```python
from build123d import *

# Parameters (mm, degrees)
F2_R     = 4.7625
F3_DEPTH = 9.525
F4_R     = 1.5875
F5_DEPTH = 20.9169


with BuildPart() as f1:
    # F0 (on Front) → F1 (revolve)
    with BuildSketch(Plane.XZ):
        with BuildLine():
            Line((0, 33.02), (0, 0))
            add(Edge.make_bspline(
                [(9.9140361241, 6.2119723298), (5.3911280841, 4.3766633401), (5.9293914696, 2.4382627623), (0, 0)],
                knots=[0.8288382909, 0.8288382909, 0.8288382909, 0.8288382909, 1, 1, 1, 1], degree=3))
            Line((9.9140361241, 6.2119723298), (9.9140361241, 13.9279487485))
            Line((9.9140361241, 13.9279487485), (9.9140361241, 21.6439251673))
            add(Edge.make_bspline(
                [(10.16, 28.857588768), (11.523254674, 26.9400200202), (10.1686139157, 23.2379404383), (9.2103585852, 22.1157759581), (9.9140361241, 21.6439251673)],
                knots=[0.1658124621, 0.1658124621, 0.1658124621, 0.1658124621, 0.2850146806, 0.3472062164, 0.3472062164, 0.3472062164, 0.3472062164], degree=3))
            add(Edge.make_bspline(
                [(0.6915654728, 33.02), (3.173352175, 32.8639093886), (8.4465738437, 31.2677125048), (10.16, 28.857588768)],
                knots=[0.0159914469, 0.0159914469, 0.0159914469, 0.0159914469, 0.1658124621, 0.1658124621, 0.1658124621, 0.1658124621], degree=3))
            Line((0.6915654728, 33.02), (0, 33.02))
        make_face()
        with BuildLine():
            Line((10.16, 33.02), (0.6915654728, 33.02))
            add(Edge.make_bspline(
                [(0.6915654728, 33.02), (3.173352175, 32.8639093886), (8.4465738437, 31.2677125048), (10.16, 28.857588768)],
                knots=[0.0159914469, 0.0159914469, 0.0159914469, 0.0159914469, 0.1658124621, 0.1658124621, 0.1658124621, 0.1658124621], degree=3))
            Line((10.16, 28.857588768), (10.16, 33.02))
        make_face()
        with BuildLine():
            Line((9.9140361241, 13.9279487485), (9.9140361241, 6.2119723298))
            add(Edge.make_bspline(
                [(31.75, 13.483504906), (30.91482321, 10.9141221863), (15.9329484904, 8.6543310681), (9.9140361241, 6.2119723298)],
                knots=[0.60106286, 0.60106286, 0.60106286, 0.60106286, 0.8288382909, 0.8288382909, 0.8288382909, 0.8288382909], degree=3))
            Line((31.75, 13.483504906), (31.75, 13.9279487485))
            Line((31.75, 13.9279487485), (9.9140361241, 13.9279487485))
        make_face()
        with BuildLine():
            Line((9.9140361241, 21.6439251673), (9.9140361241, 13.9279487485))
            Line((9.9140361241, 13.9279487485), (31.75, 13.9279487485))
            add(Edge.make_bspline(
                [(9.9140361241, 21.6439251673), (12.6387933507, 19.8168399172), (30.8403124733, 16.6836184602), (31.75, 13.9279487485)],
                knots=[0.3472062164, 0.3472062164, 0.3472062164, 0.3472062164, 0.5880222536, 0.5880222536, 0.5880222536, 0.5880222536], degree=3))
        make_face()
        with BuildLine():
            add(Edge.make_bspline(
                [(9.9140361241, 21.6439251673), (12.6387933507, 19.8168399172), (30.8403124733, 16.6836184602), (31.75, 13.9279487485)],
                knots=[0.3472062164, 0.3472062164, 0.3472062164, 0.3472062164, 0.5880222536, 0.5880222536, 0.5880222536, 0.5880222536], degree=3))
            Line((31.75, 13.9279487485), (31.75, 21.6439251673))
            Line((31.75, 21.6439251673), (9.9140361241, 21.6439251673))
        make_face()
        with BuildLine():
            add(Edge.make_bspline(
                [(31.75, 13.483504906), (30.91482321, 10.9141221863), (15.9329484904, 8.6543310681), (9.9140361241, 6.2119723298)],
                knots=[0.60106286, 0.60106286, 0.60106286, 0.60106286, 0.8288382909, 0.8288382909, 0.8288382909, 0.8288382909], degree=3))
            Line((9.9140361241, 6.2119723298), (31.75, 6.2119723298))
            Line((31.75, 6.2119723298), (31.75, 13.483504906))
        make_face()
    revolve(axis=Axis((0, 0, 16.51), (0, 0, 1)))

    # F2 (on face) → F3 (cut)
    with BuildSketch(Plane.XY.offset(33.02)):
        Circle(F2_R)
    extrude(amount=-F3_DEPTH, mode=Mode.SUBTRACT)

    # F4 (on Top) → F5 (cut)
    with BuildSketch(Plane.XY):
        Circle(F4_R)
    extrude(amount=F5_DEPTH, mode=Mode.SUBTRACT)


solid = f1.part
```
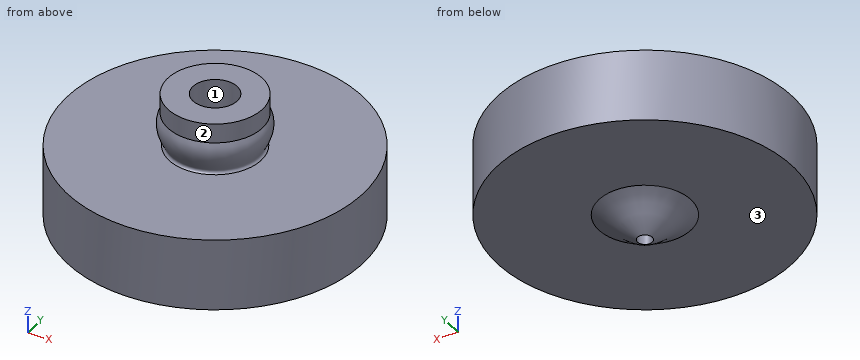
Part model, mm, in its own coordinate system. Face numbers are marked on the shaded views. Round coordinates to 2 decimals unless told otherwise and drop trailing zeros. Loops run counter-clockwise (first coordinate to the right, second up) from the corner with the lowest first, then second, coordinate; pieces in that order, holes last. Notation, with made-up numbers: (18.5, -40) -> (57.5, -40) arc R9 cw to (57.5, -30) -> close; hole circle Ø6 at (86, 42.25). An arc over 180 degrees is marked (long way). Use CSV: the item, a comma, the result in double quotes. Start each with the question number.
1) Drop flat-ended pins along their axis: P1, Ø1, axis at y = -3.5, z = 16.5, coming from the +X side; P2, Ø1, axis at x = -8, z = 8, coming from the +Y side; P3, Ø1.9, axis at x = 0, y = 0, coming from the +Z side (3 decimals). Give the stop position or say it passes through.
2) Cut at C-C, the plane x = 16. Write the cut outline in (y, z), plus the area to 3 significant figures.
3) Cut at B-B, the plane y = -19. Write the cut outline in (x, z), plus the area to 3 significant figures.
4) Pull direction X, two halves, no side cores. Call the marked faces 1, 2 and 3: +X half, -X half, draft (parallel to the pull), parting line (faces both ways), or undercut.
5) Wall check: L1, parallel to Y at x = 0, z = 30; L2, parallel to Y at x = 0, z = 10.5; L3, parallel to Z at x = 4, y = 24.5. Give the ranges that are in metal, low to high. Write a range as [from, to].
Determined:
1,P1,"stops at x = 31.61"
1,P2,"stops at y = 30.85"
1,P3,"stops at z = 23.495"
2,outline,"(-27.42, 6.21) -> (27.42, 6.21) -> (27.42, 21.64) -> (-27.42, 21.64) -> close"
2,area,"846 mm2"
3,outline,"(-25.44, 6.21) -> (25.44, 6.21) -> (25.44, 21.64) -> (-25.44, 21.64) -> close"
3,area,"785 mm2"
4,face 1,"undercut"
4,face 2,"parting line"
4,face 3,"draft"
5,L1,"y = [-10.16, -4.76], [4.76, 10.16]"
5,L2,"y = [-31.75, -1.59], [1.59, 31.75]"
5,L3,"z = [6.21, 21.64]"
